The listing builds one solid part. Answer for the finished solid, in the listing's coordinates (mm). Face numbers are marked on the shaded views. Give positions to 0.01 mm unless a question says otherwise; leave off trailing zeros. Order: outer loops, then holes, each group sorted by start corner. A loop starts at its lowest first (then second) coordinate and runs counter-clockwise, first axis right, second up. Notation, with made-up numbers: (-20.5, 65) - (-2.5, 65) arc R17 cw to (-2.5, 98) - close; hole circle Ø6 at (79.25, 0). An arc over 180 degrees is marked (long way). Answer as a JSON object with one key per item and string values. Group by question number.
Q1. The mould has two halves that part along Y. Classify the marked faces 1, 2, 3 and 4: released by +Y, released by -Y, zero draft, split by the parting line, or undercut.
Q2. A cutting plane is placed at B-B, the plane x = 29.5. Give the vertices of the cut face in (y, z), and give its area (3 significant figures).
Q3. Consider line 1 (Z direction, x = 19.5, y = 2.5); line 2 (X direction, y = -13, z = -0.95); line 3 (X direction, y = -14, z = -0.6). Determine where each line is inside the solid, lowest interval first.
Q4. Given pin 1 (1.5 mm diameter, centred on y = -15, z = 1.5, fed in from -X); pin 2 (1 mm diameter, centred on y = 0, z = 1.5, fed in from -X), each flat-ended and moving along its own axis, determine where each tip first touches the part or whether it passes through.
Q5. A cutting plane is placed at A-A, the plane y = -15. Give the vertices of the cut face in (x, z) (3 decimals), and give its area (3 significant figures).
Q6. A cutting plane is placed at C-C, the plane z = 1.05. Give the vertices of the cut face in (x, y), and give its area (3 significant figures).
Q7. A cutting plane is placed at D-D, the plane y = -19. Give the vertices of the cut face in (x, z).
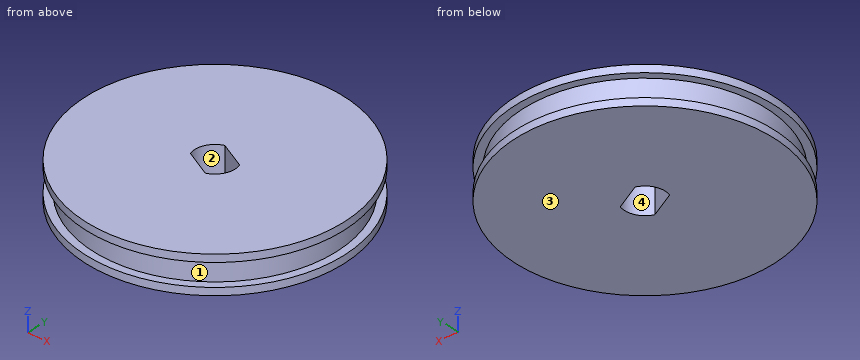
from build123d import *

# Parameters (mm, degrees)
SKETCH_1_R          = 16.25
EXTRUDE_1_DEPTH     = 1.5
SKETCH_2_R          = 17.25
EXTRUDE_2_DEPTH     = 1
CUT_EXTRUDE_1_DEPTH = 51.564922409


with BuildPart() as part:
    # 草图1 → 凸台-拉伸1 (new, symmetric)
    with BuildSketch(Plane.XY):
        with Locations((22.416532439, -13.707674049)):
            Circle(SKETCH_1_R)
    extrude(amount=EXTRUDE_1_DEPTH, both=True)

    # 草图2 → 凸台-拉伸2 (add)
    with BuildSketch(Plane.XY.offset(1.5)):
        with Locations((22.416532439, -13.707674049)):
            Circle(SKETCH_2_R)
    extrude_2 = extrude(amount=EXTRUDE_2_DEPTH)

    # 镜向1: 凸台-拉伸2 across plane
    add(extrude_2.mirror(Plane.XY))

    # 草图3 → 切除-拉伸1 (cut, through all)
    with BuildSketch(Plane.XY.offset(2.5)):
        with BuildLine():
            Line((24.98184237, -12.86554285), (21.483879203, -11.17387099))
            ThreePointArc((21.483879203, -11.17387099), (19.985859773, -12.532161228), (19.851222508, -14.549805248))
            Line((19.851222508, -14.549805248), (23.349185675, -16.241477108))
            ThreePointArc((23.349185675, -16.241477108), (24.847205105, -14.88318687), (24.98184237, -12.86554285))
        make_face()
    extrude(amount=-CUT_EXTRUDE_1_DEPTH, mode=Mode.SUBTRACT)


solid = part.part
Reply:
{
 "1": {"face 1": "split by the parting line", "face 2": "undercut", "face 3": "zero draft", "face 4": "undercut"},
 "2": {"outline": "(-29.44, -2.5) - (2.02, -2.5) - (2.02, -1.5) - (0.92, -1.5) - (0.92, 1.5) - (2.02, 1.5) - (2.02, 2.5) - (-29.44, 2.5) - (-29.44, 1.5) - (-28.33, 1.5) - (-28.33, -1.5) - (-29.44, -1.5) - close", "area": "151 mm^2"},
 "3": {"line 1": "z = -2.5 to -1.5, 1.5 to 2.5", "line 2": "x = 6.18 to 19.81, 25.02 to 38.65", "line 3": "x = 6.17 to 19.73, 25.1 to 38.66"},
 "4": {"pin 1": "stops at x = 5.18", "pin 2": "stops at x = 11.32"},
 "5": {"outline": "(5.215, -2.5) - (20.782, -2.5) - (20.782, 2.5) - (5.215, 2.5) - (5.215, 1.5) - (6.218, 1.5) - (6.218, -1.5) - (5.215, -1.5) - close; (24.787, -2.5) - (39.618, -2.5) - (39.618, -1.5) - (38.615, -1.5) - (38.615, 1.5) - (39.618, 1.5) - (39.618, 2.5) - (24.787, 2.5) - close", "area": "146 mm^2"},
 "6": {"outline": "circle Ø32.5 at (22.42, -13.71); hole (19.85, -14.55) - (23.35, -16.24) arc R2.7 ccw to (24.98, -12.87) - (21.48, -11.17) arc R2.7 ccw to start", "area": "811 mm^2"},
 "7": {"outline": "(6, -2.5) - (38.83, -2.5) - (38.83, -1.5) - (37.78, -1.5) - (37.78, 1.5) - (38.83, 1.5) - (38.83, 2.5) - (6, 2.5) - (6, 1.5) - (7.05, 1.5) - (7.05, -1.5) - (6, -1.5) - close"}
}
